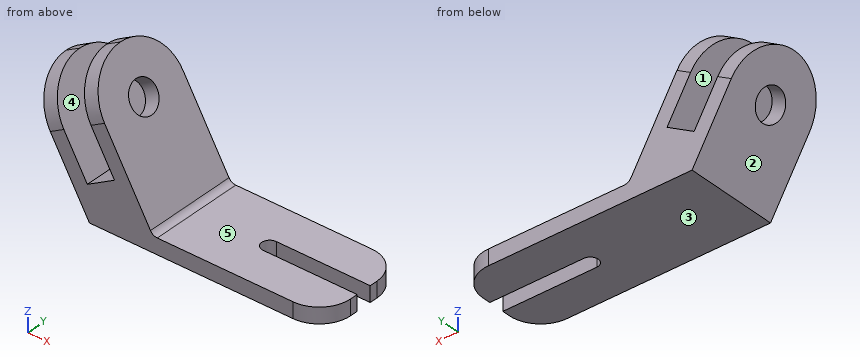
from build123d import *

# Parameters (mm, degrees)
F1_DEPTH = 60
F2_R     = 20
F4_DEPTH = 10.001
F5_R     = 29.99999
F7_D     = 20


# Not quite as in the source:
# - a fillet or chamfer is up to 0.001 mm smaller than in the source, because OpenCascade refuses the exact size


with BuildPart() as f1:
    # F0 (on Front) → F1 (new body)
    with BuildSketch(Plane.XZ):
        with BuildLine():
            Line((-40, 69.2820323028), (0, 0))
            Line((0, 0), (150, 0))
            Line((150, 0), (150, 10))
            Line((150, 10), (43.3012701892, 10))
            ThreePointArc((43.3012701892, 10), (40.8012701892, 10.6698729811), (38.9711431703, 12.5))
            Line((38.9711431703, 12.5), (-5.3589838486, 89.2820323028))
            Line((-5.3589838486, 89.2820323028), (-14.0192378865, 84.2820323028))
            Line((-14.0192378865, 84.2820323028), (15.9807621135, 32.3205080757))
            Line((15.9807621135, 32.3205080757), (-1.3397459622, 22.3205080757))
            Line((-1.3397459622, 22.3205080757), (-31.3397459622, 74.2820323028))
            Line((-31.3397459622, 74.2820323028), (-40, 69.2820323028))
        make_face()
    extrude(amount=F1_DEPTH)

    # F2
    f2_edges = [f1.edges().sort_by_distance(p)[0] for p in [
        (150, 0, 5),
        (150, -60, 5),
    ]]
    fillet(f2_edges, radius=F2_R)

    # F3 (on face) → F4 (cut, through all)
    with BuildSketch(Plane.XY.offset(10)):
        with BuildLine():
            ThreePointArc((90, -35), (93.5355339059, -33.5355339059), (95, -30))
            ThreePointArc((95, -30), (93.5818777161, -26.5114255022), (90.1319391892, -25.0017410981))
            ThreePointArc((90.1319391892, -25.0017410981), (85.0004352935, -29.9340246617), (90, -35))
        make_face()
        with BuildLine():
            ThreePointArc((90.1319391892, -25.0017410981), (93.5818777161, -26.5114255022), (95, -30))
            ThreePointArc((95, -30), (93.5355339059, -33.5355339059), (90, -35))
            Line((90, -35), (150, -35))
            Line((150, -35), (150, -25.0017410981))
            Line((150, -25.0017410981), (90.1319391892, -25.0017410981))
        make_face()
    extrude(amount=-F4_DEPTH, mode=Mode.SUBTRACT)

    # F5 (radius 30 in the source; OpenCascade refuses exactly that, so slightly less here)
    f5_edges = [f1.edges().sort_by_distance(p)[0] for p in [
        (-9.689111, -60, 86.782032),
        (-9.689111, 0, 86.782032),
        (-35.669873, -60, 71.782032),
        (-35.669873, 0, 71.782032),
    ]]
    fillet(f5_edges, radius=F5_R)

    # F7 (through all)
    with Locations(Plane(origin=(34.6410161514, 0, 20), x_dir=(0, 1, 0), z_dir=(0.8660254038, 0, 0.5))):
        with Locations((-30, 50)):
            Hole(F7_D / 2)


solid = f1.part
Geometry: final body of the model. Coordinates: model frame, mm. Face numbers are marked on the shaded views. A direction names the side the tool comes from. Give positions to 0.01 mm unless a question says otherwise; leave off trailing zeros. Order: outer loops, then holes, each group sorted by start corner. A loop starts at its lowest first (then second) coordinate and runs counter-clockwise, first axis right, second up. Notation, with made-up numbers: (54, 48) -> (98, 48) arc R14 cw to (98, 64) -> close; hole circle Ø10 at (58.5, 53.5). An arc over 180 degrees is marked (long way). Write each question's results on one line, items separated by ' | '.
1) Cut plane D-D (y = -53). Output: boundary loops of the cut face in (x, z).
Geometry says:
outline: (-34.63, 59.98) -> (0, 0) -> (145.2, 0) -> (145.2, 10) -> (43.3, 10) arc R5 cw to (38.97, 12.5) -> (0.01, 79.98) -> (-8.65, 74.98) -> (15.98, 32.32) -> (-1.34, 22.32) -> (-25.97, 64.98) -> close
2) Cut plane A-A (x = 120.5). Output: boundary loops of the cut face in (y, z), and give its area (3 significant figures).
Geometry says:
outline: (-60, 0) -> (-35, 0) -> (-35, 10) -> (-60, 10) -> close; (-25, 0) -> (0, 0) -> (0, 10) -> (-25, 10) -> close | area: 500 mm²
3) Set-up query: the marked faces 1 and 2. Return all of +Z, -Z, +X, -X, +Y, -Y with unobstructed straight access to the full face (end or side cutting, diameter ignored); none if empty.
Geometry says:
face 1: +Y, -Y | face 2: -Z, -X, +Y, -Y
4) Draft query along Z for the marked faces 3, 4 and 5. Return one class per face: released by +Z, released by -Z, zero draft, split by the parting line, or undercut.
Geometry says:
face 3: released by -Z | face 4: undercut | face 5: released by +Z
5) Cut plane C-C (x = 75). Output: boundary loops of the cut face in (y, z).
Geometry says:
outline: (-60, 0) -> (0, 0) -> (0, 10) -> (-60, 10) -> close
6) Line query: line 1 along Y through (x, z) = (-21, 45); line 2 along Z through (x, y) = (96.5, -35.5); line 3 along X through (y, z) = (-55, 46). Output: solid intervals per line, ascending.
Geometry says:
line 1: y = -60 to -39.99, -20.01 to 0 | line 2: z = 0 to 10 | line 3: x = -26.56 to -15.01, 8.08 to 19.63
7) First-contact query: pin 1 Ø12 at (x, y) = (113, -37) entering from +Z; pin 2 Ø10 at (x, z) = (10, 78) entering from -Y; pin 3 Ø6 at (y, z) = (-19, 61) entering from +X; pin 4 Ø1.5 at (y, z) = (-27.5, 23.5) entering from +X. Flat tips, straight axial feed; report the tip coordinate or a pass-through.
Geometry says:
pin 1: stops at z = 10 | pin 2: passes through | pin 3: stops at x = 12.7 | pin 4: stops at x = 33.05
8) Cut plane B-B (y = -27.5). Output: boundary loops of the cut face in (x, z), and give its area (3 significant figures).
Geometry says:
outline: (-39.95, 69.19) -> (-29.84, 51.69) -> (-21.18, 56.69) -> (-31.29, 74.19) -> close; (-20.16, 34.92) -> (0, 0) -> (85.67, 0) -> (85.67, 10) -> (43.3, 10) arc R5 cw to (38.97, 12.5) -> (14.48, 54.92) -> (5.82, 49.92) -> (15.98, 32.32) -> (-1.34, 22.32) -> (-11.5, 39.92) -> close; (-13.97, 84.19) -> (-3.86, 66.69) -> (4.8, 71.69) -> (-5.31, 89.19) -> close | area: 2,500 mm²
